from build123d import *

# Parameters (mm, degrees)
SKETCH1_W            = 50
SKETCH1_H            = 180
BOSS_EXTRUDE1_DEPTH  = 8
M5_CLEARANCE_HOLE1_D = 5.3
M6_CLEARANCE_HOLE1_D = 6.4


with BuildPart() as part:
    # Sketch1 → Boss-Extrude1 (new body)
    with BuildSketch(Plane.XY):
        Rectangle(SKETCH1_W, SKETCH1_H)
    extrude(amount=BOSS_EXTRUDE1_DEPTH)

    # M5 Clearance Hole1 (through all)
    with Locations(Plane.XY.offset(8)):
        with Locations((-15, 45), (-15, -45), (15, -45), (15, 45), (-15, 75), (-15, -75), (15, -75), (15, 75)):
            Hole(M5_CLEARANCE_HOLE1_D / 2)

    # M6 Clearance Hole1 (through all)
    with Locations(Plane.XY.offset(8)):
        with Locations((-6.5, 23), (-6.5, -23), (6.5, -23), (6.5, 23)):
            Hole(M6_CLEARANCE_HOLE1_D / 2)


solid = part.part
Input: part model. Units: mm. Frame: model coordinates. Coordinates: 2 decimals unless noted, no trailing zeros. Loops run counter-clockwise (first coordinate to the right, second up) from the corner with the lowest first, then second, coordinate; pieces in that order, holes last. Notation, with made-up numbers: (-31.5, -33.75) - (26.5, -33.75) arc R23 ccw to (26.5, -10.75) - close; hole circle Ø8 at (-19.75, 35.5). An arc over 180 degrees is marked (long way). Answer in a Markdown table with one row per item. Add a question column.
Item 1: Line query: line 1 along Y through (x, z) = (15, 2); line 2 along Y through (x, z) = (6.5, 2.5); line 3 along Y through (x, z) = (-14, 1). Output: solid intervals per line, ascending. Write a range as [from, to].
Item 2: Section query D-D on x = -6.5. Return the cut outline in (y, z).
Item 3: Section query C-C on y = -23. Return the cut outline in (x, z).
Item 4: Mould query, pull axis X, two halves, no side actions, for faces 1 (the cylindrical face through (5.023, -25.839, 3.944)), 2 (the flat face through (25, -1, 4)), 3 (the flat face through (0, 1, 8)). Classes: released by +X, released by -X, zero draft, split by the parting line, or undercut.
Item 5: Section query B-B on x = -15. Return the cut outline in (y, z), then the cut area to 3 significant figures.
Item 6: Section query A-A on z = 5.5. State how many separate pieces and enclosed holes the cut face has, then the cut area to 3 significant figures.
Recorded:
| question | item | result |
|---|---|---|
| 1 | line 1 | [-90, -77.65], [-72.35, -47.65], [-42.35, 42.35], [47.65, 72.35], [77.65, 90] |
| 1 | line 2 | [-90, -26.2], [-19.8, 19.8], [26.2, 90] |
| 1 | line 3 | [-90, -77.45], [-72.55, -47.45], [-42.55, 42.55], [47.45, 72.55], [77.45, 90] |
| 2 | outline | (-90, 0) - (-26.2, 0) - (-26.2, 8) - (-90, 8) - close; (-19.8, 0) - (19.8, 0) - (19.8, 8) - (-19.8, 8) - close; (26.2, 0) - (90, 0) - (90, 8) - (26.2, 8) - close |
| 3 | outline | (-25, 0) - (-9.7, 0) - (-9.7, 8) - (-25, 8) - close; (-3.3, 0) - (3.3, 0) - (3.3, 8) - (-3.3, 8) - close; (9.7, 0) - (25, 0) - (25, 8) - (9.7, 8) - close |
| 4 | face 1 | undercut |
| 4 | face 2 | released by +X |
| 4 | face 3 | zero draft |
| 5 | outline | (-90, 0) - (-77.65, 0) - (-77.65, 8) - (-90, 8) - close; (-72.35, 0) - (-47.65, 0) - (-47.65, 8) - (-72.35, 8) - close; (-42.35, 0) - (42.35, 0) - (42.35, 8) - (-42.35, 8) - close; (47.65, 0) - (72.35, 0) - (72.35, 8) - (47.65, 8) - close; (77.65, 0) - (90, 0) - (90, 8) - (77.65, 8) - close |
| 5 | area | 1,270 mm^2 |
| 6 | separate pieces | 1 |
| 6 | enclosed holes | 12 |
| 6 | area | 8,690 mm^2 |
